from build123d import *

# Parameters (mm, degrees)
SKETCH1_R           = 1.6
BOSS_EXTRUDE1_DEPTH = 3
SKETCH2_W           = 10
SKETCH2_H           = 10
BOSS_EXTRUDE2_DEPTH = 42
CHAMFER1_SIZE       = 5
SKETCH3_R           = 2.1
CUT_EXTRUDE1_DEPTH  = 52
SKETCH4_R           = 2.65
CUT_EXTRUDE2_DEPTH  = 0.5
SKETCH11_W          = 6
SKETCH11_H          = 3
BOSS_EXTRUDE7_DEPTH = 8
SKETCH12_R          = 1.2
CUT_EXTRUDE5_DEPTH  = 72.139584736
FILLET1_R           = 2
SKETCH13_W          = 2
SKETCH13_H          = 3
BOSS_EXTRUDE8_DEPTH = 10
SKETCH14_W          = 2
SKETCH14_H          = 10
BOSS_EXTRUDE9_DEPTH = 3
SKETCH15_R          = 1
CUT_EXTRUDE6_DEPTH  = 3


with BuildPart() as part:
    # Sketch1 → Boss-Extrude1 (new body)
    with BuildSketch(Plane(origin=(0, 0, 0), x_dir=(1, 0, 0), z_dir=(0, 1, 0))):
        Polygon((-6.512396694, 9.685950413), (1.487603306, 9.685950413), (26.487603306, 9.685950413), (26.487603306, -40.314049587), (1.487603306, -40.314049587), (-6.512396694, -40.314049587), align=None)
        with Locations(Location((-1.962396694, -35.764049587, 0), (0, 0, 270))):
            Circle(SKETCH1_R, mode=Mode.SUBTRACT)
        with Locations(Location((-1.962396694, 5.135950413, 0), (0, 0, 270))):
            Circle(SKETCH1_R, mode=Mode.SUBTRACT)
    extrude(amount=BOSS_EXTRUDE1_DEPTH)

    # Sketch2 → Boss-Extrude2 (add)
    with BuildSketch(Plane(origin=(0, 3, 0), x_dir=(1, 0, 0), z_dir=(0, 1, 0))):
        with Locations((21.487603306, -35.314049587)):
            Rectangle(SKETCH2_W, SKETCH2_H)
        with Locations((21.487603306, 4.685950413)):
            Rectangle(SKETCH2_W, SKETCH2_H)
    extrude(amount=BOSS_EXTRUDE2_DEPTH)

    # Chamfer1
    chamfer1_edges = [part.edges().sort_by_distance(p)[0] for p in [
        (21.487603306, 3, 30.314049587),
        (16.487603306, 3, 35.314049587),
        (16.487603306, 3, -4.685950413),
        (21.487603306, 3, 0.314049587),
    ]]
    chamfer(chamfer1_edges, length=CHAMFER1_SIZE)

    # Sketch3 → Cut-Extrude1 (cut)
    with BuildSketch(Plane(origin=(0, 45, 0), x_dir=(1, 0, 0), z_dir=(0, 1, 0))):
        with Locations(Location((22.537603306, -36.364049587, 0), (0, 0, 270))):
            Circle(SKETCH3_R)
        with Locations(Location((22.537603306, 5.735950413, 0), (0, 0, 270))):
            Circle(SKETCH3_R)
    extrude(amount=-CUT_EXTRUDE1_DEPTH, mode=Mode.SUBTRACT)

    # Sketch4 → Cut-Extrude2 (cut)
    with BuildSketch(Plane(origin=(0, 45, 0), x_dir=(1, 0, 0), z_dir=(0, 1, 0))):
        with Locations(Location((22.537603306, -36.364049587, 0), (0, 0, 270))):
            Circle(SKETCH4_R)
        with Locations(Location((22.537603306, 5.735950413, 0), (0, 0, 270))):
            Circle(SKETCH4_R)
    cut_extrude2 = extrude(amount=-CUT_EXTRUDE2_DEPTH, mode=Mode.SUBTRACT)

    # Mirror1: Cut-Extrude2 across plane
    add(cut_extrude2.mirror(Plane(origin=(0, 22.5, 0), x_dir=(0, 0, 1), z_dir=(0, -1, 0))), mode=Mode.SUBTRACT)

    # Sketch11 → Boss-Extrude7 (add)
    with BuildSketch(Plane.XY.offset(40.314049587)):
        with Locations((21.487603306, 43.5)):
            Rectangle(SKETCH11_W, SKETCH11_H)
        with Locations((21.487603306, 1.5)):
            Rectangle(SKETCH11_W, SKETCH11_H)
    extrude(amount=BOSS_EXTRUDE7_DEPTH)

    # Sketch12 → Cut-Extrude5 (cut, through all)
    with BuildSketch(Plane.XZ):
        with Locations(Location((21.487603306, 45.314049587, 0), (0, 0, 270))):
            Circle(SKETCH12_R)
    extrude(amount=-CUT_EXTRUDE5_DEPTH, mode=Mode.SUBTRACT)

    # Fillet1
    fillet1_edges = [part.edges().sort_by_distance(p)[0] for p in [
        (18.487603306, 43.5, 40.314049587),
        (18.487603306, 1.5, 40.314049587),
        (24.487603306, 1.5, 40.314049587),
    ]]
    fillet(fillet1_edges, radius=FILLET1_R - 0.0001)  # a hair under: the kernel refuses the full size
    fillet1_2_edges = [part.edges().sort_by_distance(p)[0] for p in [
        (18.487603306, 43.5, 48.314049587),
        (24.487603306, 1.5, 48.314049587),
        (18.487603306, 1.5, 48.314049587),
    ]]
    fillet(fillet1_2_edges, radius=FILLET1_R)

    # Sketch13 → Boss-Extrude8 (add)
    with BuildSketch(Plane.XY.offset(40.314049587)):
        with Locations((25.487603306, 43.5)):
            Rectangle(SKETCH13_W, SKETCH13_H)
    extrude(amount=BOSS_EXTRUDE8_DEPTH)

    # Sketch14 → Boss-Extrude9 (add)
    with BuildSketch(Plane.XZ.offset(-42)):
        with Locations((25.487603306, 45.314049587)):
            Rectangle(SKETCH14_W, SKETCH14_H)
    extrude(amount=BOSS_EXTRUDE9_DEPTH)

    # Sketch15 → Cut-Extrude6 (cut)
    with BuildSketch(Plane(origin=(26.487603306, 0, 0), x_dir=(0, 0, -1), z_dir=(1, 0, 0))):
        with Locations((-48.614049587, 42.5)):
            Circle(SKETCH15_R)
    extrude(amount=-CUT_EXTRUDE6_DEPTH, mode=Mode.SUBTRACT)


solid = part.part
Source: CAD feature listing. Evaluate the final solid. Frame: model axes, mm. A direction names the side the tool comes from. Coordinates: 2 decimals unless noted, no trailing zeros. Loops run counter-clockwise (first coordinate to the right, second up) from the corner with the lowest first, then second, coordinate; pieces in that order, holes last. Notation, with made-up numbers: (17, 29) - (53, 29) arc R3 cw to (53, 33) - close; hole circle Ø4 at (71.5, 49). An arc over 180 degrees is marked (long way). One line per item, written item: value. Start each with the question number.
1. Ray query, L1, parallel to X at y = 38.5, z = -6; L2, parallel to Y at x = 22, z = 42.5; L3, parallel to Y at x = 3.5, z = 28.5. Return the intervals inside material, ascending.
2. Set-up query: faces 1 (the flat face through (18, 19, 40.314)), 2 (the cylindrical face through (22.654, 44.754, 33.717)), 3 (the cylindrical face through (25.34, 42.8, 47.66)), 4 (the flat face through (22, 44, 48.314)), 5 (the flat face through (20.549, 5.535, 27.849)). Return all of +Z, -Z, +X, -X, +Y, -Y with unobstructed straight access to the full face (end or side cutting, diameter ignored); none if empty.
3. Section A-A (y = 14.5). Return the cut outline in (x, z).
4. Section B-B (z = 13.5). Return the cut outline in (x, y), and give its area (3 significant figures).
5. Contact query for flat-ended pins moving along their axis: P1, Ø1.9, axis at x = 21.49, z = 45.31, coming from the +Y side; P2, Ø1.8, axis at y = 43, z = 47, coming from the -X side; P3, Ø1, axis at x = 7.5, z = 9.5, coming from the +Y side; P4, Ø1.6, axis at x = 23.5, z = -4.5, coming from the -Y side. Output: stop coordinate, or through.
6. Mould query, pull axis X, two halves, no side actions, for faces 6 (the cylindrical face through (25.089, 1.521, 40.884)), 7 (the cylindrical face through (-3.382, 1.479, 36.502)), 8 (the flat face through (21, 26, 0.314)). Classes: pulls with the +X half, pulls with the -X half, needs draft (parallel to the pull), parting line crosses it, or undercut.
7. Section C-C (x = 3). Return the cut outline in (y, z).
Verdict:
1. L1: x = 16.49 to 20.45, 24.62 to 26.49
1. L2: y = 0 to 3, 42 to 45
1. L3: y = 0 to 3
2. face 1: +Z, -X
2. face 2: +Y
2. face 3: +X
2. face 4: +Z, -X, +Y, -Y
2. face 5: +X, -X, +Y
3. outline: (16.49, -9.69) - (26.49, -9.69) - (26.49, 0.31) - (16.49, 0.31) - close; (16.49, 30.31) - (26.49, 30.31) - (26.49, 40.31) - (16.49, 40.31) - close; hole circle Ø4.2 at (22.54, -5.74); hole circle Ø4.2 at (22.54, 36.36)
4. outline: (-6.51, 0) - (26.49, 0) - (26.49, 3) - (-6.51, 3) - close
4. area: 99.0 mm2
5. P1: passes through
5. P2: stops at x = 18.49
5. P3: stops at y = 3
5. P4: stops at y = 0.5
6. face 6: pulls with the +X half
6. face 7: undercut
6. face 8: needs draft
7. outline: (0, -9.69) - (3, -9.69) - (3, 40.31) - (0, 40.31) - close
